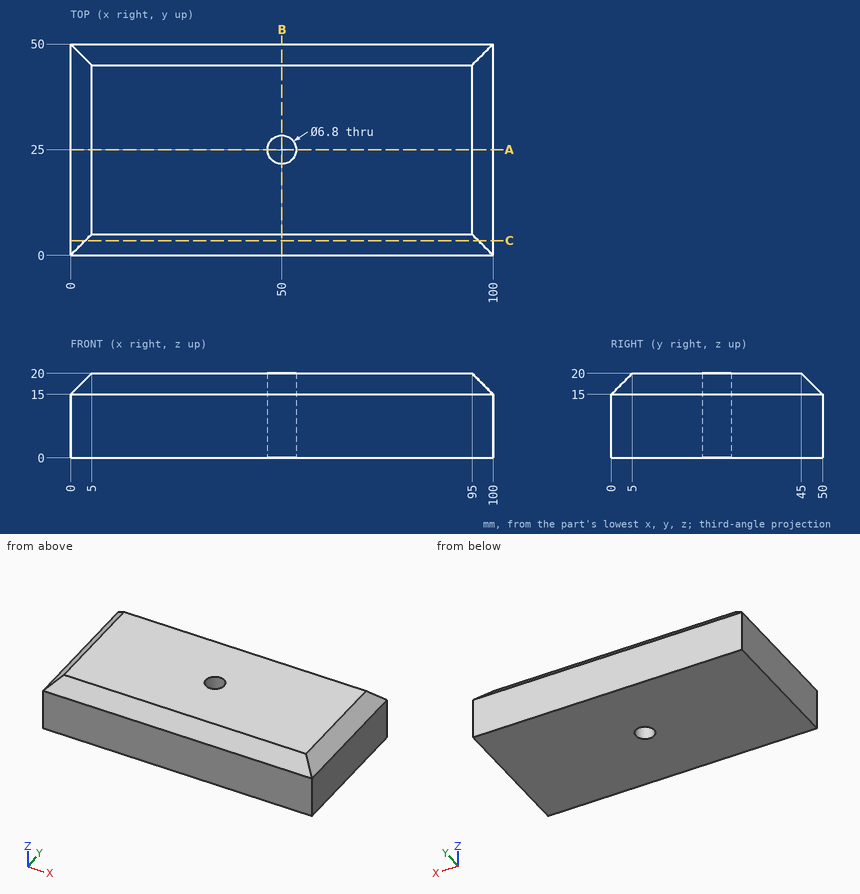
Job drawing, mm, ordinate dimensions from the low corner. One solid piece. Coordinates: 2 decimals unless noted, no trailing zeros. Write each loop counter-clockwise with the first axis right and the second up, starting at its lowest first coordinate (ties: lowest second). Pieces come first, ordered by that corner, then holes. Notation, with made-up numbers: (79, 48.5) - (103, 48.5) arc R15 cw to (103, 62.5) - close; hole circle Ø3 at (-28.5, 3). An arc over 180 degrees is marked (long way). Use a Markdown table: item, result. Add a question column.
Item 1: Band-saw the part on C-C, the plane y = 3.5. Give the cut face in (x, z).
Item 2: Band-saw the part on A-A, the plane y = 25. Give the cut face in (x, z), and give its area (3 significant figures).
Item 3: Band-saw the part on B-B, the plane x = 50. Give the cut face in (y, z).
Item 4: Drill centre lines: L1, parallel to Y at x = 50, z = 8.5; L2, parallel to Y at x = 48, z = 15.5; L3, parallel to Y at x = 64.5, z = 15.25. Where is each one in solid material? Low to high. Write a range as from..to.
Numbers:
| question | item | result |
|---|---|---|
| 1 | outline | (0, 0) - (100, 0) - (100, 15) - (96.5, 18.5) - (3.5, 18.5) - (0, 15) - close |
| 2 | outline | (0, 0) - (46.6, 0) - (46.6, 20) - (5, 20) - (0, 15) - close; (53.4, 0) - (100, 0) - (100, 15) - (95, 20) - (53.4, 20) - close |
| 2 | area | 1,840 mm2 |
| 3 | outline | (0, 0) - (21.6, 0) - (21.6, 20) - (5, 20) - (0, 15) - close; (28.4, 0) - (50, 0) - (50, 15) - (45, 20) - (28.4, 20) - close |
| 4 | L1 | 0..21.6, 28.4..50 |
| 4 | L2 | 0.5..22.25, 27.75..49.5 |
| 4 | L3 | 0.25..49.75 |
